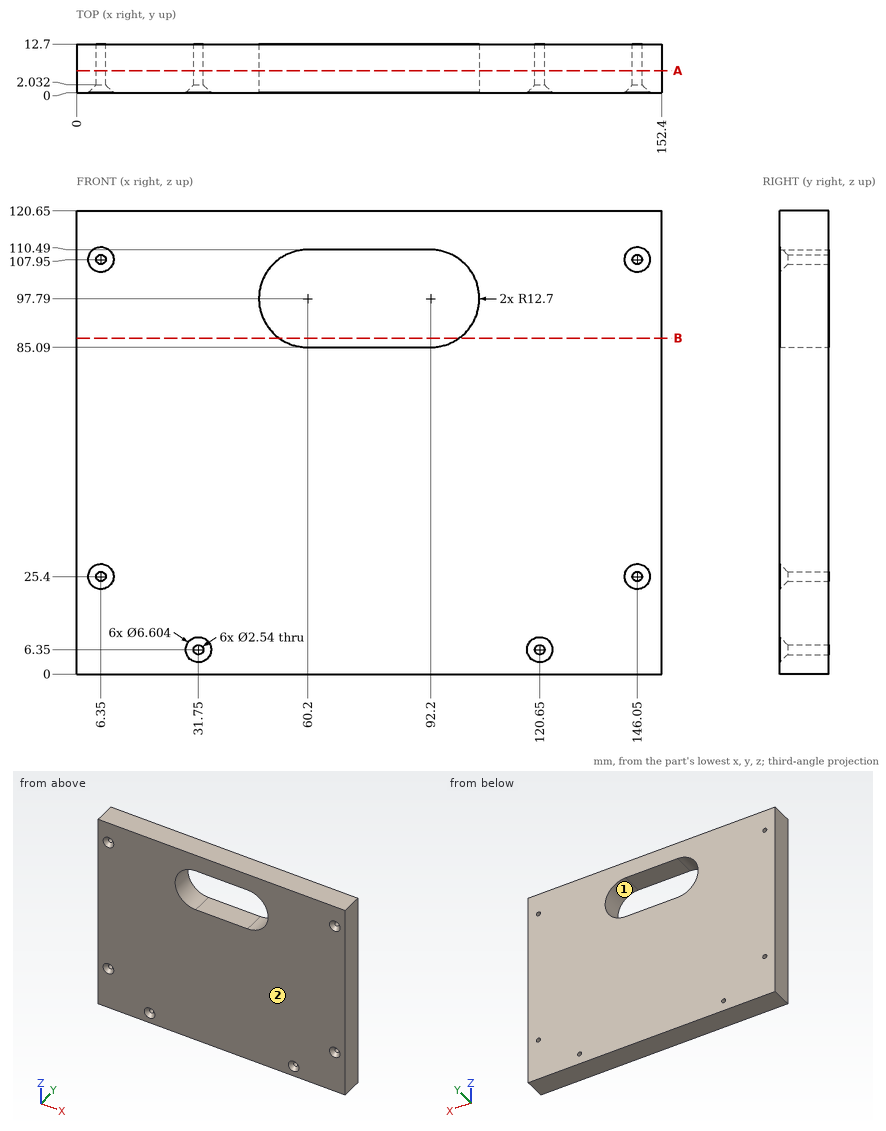
Check sheet for the drawn part. Datum: minimum x, y, z corner. Units: mm. A direction names the side the tool comes from. Coordinates: 2 decimals unless noted, no trailing zeros. Write each loop counter-clockwise with the first axis right and the second up, starting at its lowest first coordinate (ties: lowest second). Pieces come first, ordered by that corner, then holes. Notation, with made-up numbers: M 56,77.25 L 82,77.25 A19 cw 82,98.25 Z; hole C 78.5,-13 d7. An arc over 180 degrees is marked long. One line per item, written item: value.
Item 1: Gauge pin test, flat ends, axial feed: pin 1 Ø1.5 at (x, z) = (6.35, 25.4) entering from +Y; pin 2 Ø4 at (x, z) = (146.05, 107.95) entering from -Y. Record the tip position at first contact, or that the pin passes through.
Check sheet entries:
pin 1: passes through
pin 2: stops at y = 1.3
Item 2: Access from +Z, -Z, +X, -X, +Y, -Y to the whole of each face (thin tool, end or side, straight path). Record for the marked faces 1 and 2.
Check sheet entries:
face 1: +Y, -Y
face 2: +Z, -Z, +X, -X, -Y
Item 3: Scan lines: line 1 along Z through (x, y) = (6.35, 8); line 2 along X through (y, z) = (9, 107.95); line 3 along Z through (x, y) = (145.5, 5.25). Record each from-to range of solid material in increasing order.
Check sheet entries:
line 1: z = 0 to 24.13, 26.67 to 106.68, 109.22 to 120.65
line 2: x = 0 to 5.08, 7.62 to 52.58, 99.82 to 144.78, 147.32 to 152.4
line 3: z = 0 to 24.26, 26.54 to 106.81, 109.09 to 120.65
Item 4: Section check B-B, the plane z = 87.5. Record the boundary of the cut face in (x, y).
Check sheet entries:
outline: M 0,0 L 52.76,0 L 52.76,12.7 L 0,12.7 Z; M 99.64,0 L 152.4,0 L 152.4,12.7 L 99.64,12.7 Z
Item 5: Section check A-A, the plane y = 5.75. Record the boundary of the cut face in (x, z).
Check sheet entries:
outline: M 0,0 L 152.4,0 L 152.4,120.65 L 0,120.65 Z; hole C 6.35,25.4 d2.54; hole C 6.35,107.95 d2.54; hole C 31.75,6.35 d2.54; hole M 60.2,85.09 L 92.2,85.09 A12.7 ccw 92.2,110.49 L 60.2,110.49 A12.7 ccw Z; hole C 120.65,6.35 d2.54; hole C 146.05,25.4 d2.54; hole C 146.05,107.95 d2.54
